```python
from build123d import *

# Parameters (mm, degrees)
F0_W      = 198
F0_H      = 198
F1_DEPTH  = 30
F2_W      = 138
F2_H      = 138
F3_DEPTH  = 30
F4_W      = 94
F4_H      = 94
F5_DEPTH  = 30
F6_R      = 4
F7_DEPTH  = 215
F9_DEPTH  = 215
F11_DEPTH = 25
F13_DEPTH = 25
F15_DEPTH = 25
F17_DEPTH = 25
F18_R     = 33.2568147927
F19_DEPTH = 6
F20_R     = 105
F20_R_2   = 33.2568147927
F21_DEPTH = 170
F21_TAPER = 10


with BuildPart() as f1:
    # F0 (on Top) → F1 (new body)
    with BuildSketch(Plane.XY):
        with Locations((99, 99)):
            Rectangle(F0_W, F0_H)
    extrude(amount=F1_DEPTH)

    # F2 (on face) → F3 (join)
    with BuildSketch(Plane.XY.offset(30)):
        with Locations((99, 99)):
            Rectangle(F2_W, F2_H)
    extrude(amount=F3_DEPTH)

    # F4 (on face) → F5 (join)
    with BuildSketch(Plane.XY.offset(60)):
        with Locations((99, 99)):
            Rectangle(F4_W, F4_H)
    extrude(amount=F5_DEPTH)

    # F6 (on face) → F7 (join)
    with BuildSketch(Plane.XY.offset(90)):
        with Locations((99, 99)):
            Circle(F6_R)
    extrude(amount=F7_DEPTH)

    # F8 (on face) → F9 (join)
    with BuildSketch(Plane.XY.offset(90)):
        Polygon((86.6256313292, 111.3743686708), (65.4124278936, 132.5875721064), (60.1091270347, 127.2842712475), (81.3223304703, 106.0710678119), align=None)
        Polygon((70.7157287525, 137.8908729653), (65.4124278936, 132.5875721064), (86.6256313292, 111.3743686708), (91.9289321881, 116.6776695297), align=None)
        Polygon((127.2842712475, 137.8908729653), (106.0710678119, 116.6776695297), (111.3743686708, 111.3743686708), (132.5875721064, 132.5875721064), align=None)
        Polygon((132.5875721064, 132.5875721064), (111.3743686708, 111.3743686708), (116.6776695297, 106.0710678119), (137.8908729653, 127.2842712475), align=None)
        Polygon((137.8908729653, 70.7157287525), (116.6776695297, 91.9289321881), (111.3743686708, 86.6256313292), (132.5875721064, 65.4124278936), align=None)
        Polygon((111.3743686708, 86.6256313292), (106.0710678119, 81.3223304703), (127.2842712475, 60.1091270347), (132.5875721064, 65.4124278936), align=None)
        Polygon((91.9289321881, 81.3223304703), (86.6256313292, 86.6256313292), (65.4124278936, 65.4124278936), (70.7157287525, 60.1091270347), align=None)
        Polygon((86.6256313292, 86.6256313292), (81.3223304703, 91.9289321881), (60.1091270347, 70.7157287525), (65.4124278936, 65.4124278936), align=None)
    extrude(amount=F9_DEPTH)

    # F10 (on face) → F11 (cut)
    with BuildSketch(Plane(origin=(5.3033008589, -5.3033008589, 0), x_dir=(0.7071067812, 0.7071067812, 0), z_dir=(0.7071067812, -0.7071067812, 0))):
        with BuildLine():
            Line((122.5071426749, 90), (122.5071426749, 305))
            ThreePointArc((122.5071426749, 305), (108.1413524776, 197.5), (122.5071426749, 90))
        make_face()
        with BuildLine():
            ThreePointArc((100.5295589566, 90), (93.5255146575, 197.840533222), (107.5071426749, 305))
            Line((107.5071426749, 305), (92.5071426749, 305))
            Line((92.5071426749, 305), (92.5071426749, 90))
            Line((92.5071426749, 90), (100.5295589566, 90))
        make_face()
    extrude(amount=-F11_DEPTH, mode=Mode.SUBTRACT)

    # F12 (on face) → F13 (cut)
    with BuildSketch(Plane(origin=(104.3033008589, 104.3033008589, 0), x_dir=(-0.7071067812, 0.7071067812, 0), z_dir=(0.7071067812, 0.7071067812, 0))):
        with BuildLine():
            Line((17.5, 305), (17.5, 90))
            ThreePointArc((17.5, 90), (28.9852035419, 197.5), (17.5, 305))
        make_face()
        with BuildLine():
            ThreePointArc((32.5, 305), (46.5125090054, 197.8568495491), (39.962310344, 90))
            Line((39.962310344, 90), (47.5, 90))
            Line((47.5, 90), (47.5, 305))
            Line((47.5, 305), (32.5, 305))
        make_face()
    extrude(amount=-F13_DEPTH, mode=Mode.SUBTRACT)

    # F14 (on face) → F15 (cut)
    with BuildSketch(Plane(origin=(5.3033008589, -5.3033008589, 0), x_dir=(0.7071067812, 0.7071067812, 0), z_dir=(0.7071067812, -0.7071067812, 0))):
        with BuildLine():
            ThreePointArc((172.5071426749, 305), (186.2558070406, 197.8608173435), (180.4356426001, 90))
            Line((180.4356426001, 90), (187.5071426749, 90))
            Line((187.5071426749, 90), (187.5071426749, 305))
            Line((187.5071426749, 305), (172.5071426749, 305))
        make_face()
        with BuildLine():
            Line((157.5071426749, 305), (157.5071426749, 90))
            ThreePointArc((157.5071426749, 90), (167.3211795092, 197.5), (157.5071426749, 305))
        make_face()
    extrude(amount=-F15_DEPTH, mode=Mode.SUBTRACT)

    # F16 (on face) → F17 (cut)
    with BuildSketch(Plane(origin=(104.3033008589, 104.3033008589, 0), x_dir=(-0.7071067812, 0.7071067812, 0), z_dir=(0.7071067812, 0.7071067812, 0))):
        with BuildLine():
            ThreePointArc((-42.129099369, 90), (-46.2365441061, 197.8995849807), (-32.5, 305))
            Line((-32.5, 305), (-47.5, 305))
            Line((-47.5, 305), (-47.5, 90))
            Line((-47.5, 90), (-42.129099369, 90))
        make_face()
        with BuildLine():
            Line((-17.5, 90), (-17.5, 305))
            ThreePointArc((-17.5, 305), (-27.2443014962, 197.5), (-17.5, 90))
        make_face()
    extrude(amount=-F17_DEPTH, mode=Mode.SUBTRACT)

    # F18 (on face) → F19 (join)
    with BuildSketch(Plane.XY.offset(305)):
        with Locations((99, 99)):
            Circle(F18_R)
    extrude(amount=F19_DEPTH)

    # F20 (on face) → F21 (join)
    with BuildSketch(Plane.XY.offset(311)):
        with Locations((99, 99)):
            Circle(F20_R)
        with Locations((99, 99)):
            Circle(F20_R_2, mode=Mode.SUBTRACT)
        with Locations((99, 99)):
            Circle(F20_R_2)
    extrude(amount=F21_DEPTH, taper=F21_TAPER)


solid = f1.part
```
Check sheet for the modelled part. Datum: model origin and axes. Units: mm. A direction names the side the tool comes from. Give positions to 0.01 mm unless a question says otherwise; leave off trailing zeros. Write each loop counter-clockwise with the first axis right and the second up, starting at its lowest first coordinate (ties: lowest second). Pieces come first, ordered by that corner, then holes. Notation, with made-up numbers: (41.25, 78.25) - (83.25, 78.25) arc R28 cw to (83.25, 102.25) - close; hole circle Ø4 at (-26, 47). An arc over 180 degrees is marked (long way). Answer as a JSON object with one key per item and string values. Group by question number.
1) Sectioned sample at A-A (z = 200). Record the cut outline in (x, y).
2) Access from +Z, -Z, +X, -X, +Y, -Y to the whole of each face (thin tool, end or side, straight path). Record for faces 4 (the face through (98, 146, 75)), 5 (the face through (0, 98, 15)), 6 (the face through (98, 52, 75)), 7 (the face through (76.54, 76.4, 199.02)).
3) Sectioned sample at B-B (z = 414). Record the cut outline in (x, y), then the cut area to 3 significant figures.
4) Release check for a two-part mould opening along Z. For faces 1 (the face through (198, 98, 15)), 2 (the face through (98, 100, 0)), 3 (the face through (68.817, 79.424, 195.995)) record: pulls with the +Z half, pulls with the -Z half, needs draft (parallel to the pull), parting line crosses it, or undercut.
5) Depth check by flat-ended pin: P1, Ø9, axis at y = 91, z = 68.5, coming from the +X side; P2, Ø4, axis at y = 124.5, z = 341.5, coming from the +X side; P3, Ø9, axis at y = 109.5, z = 42.5, coming from the -X side. Enter the tip coordinate at first touch or a pass-through.
6) Thickness scan on probe 1 along Z at (x, y) = (51.5, 137.5); probe 2 along Z at (x, y) = (63, 60.5); probe 3 along X at (y, z) = (108, 63). Record the ranges inside material, lowest first. Write a range as from..to.
Geometry results:
{
 "1": {"outline": "(60.86, 126.53) - (73.21, 114.19) - (83.81, 124.79) - (71.47, 137.14) - close; (60.88, 71.49) - (71.49, 60.88) - (81.78, 71.17) - (71.17, 81.78) - close; circle Ø8 at (99, 99); (112.96, 74.44) - (126.32, 61.07) - (136.93, 71.68) - (123.56, 85.04) - close; (113.01, 123.61) - (123.61, 113.01) - (136.95, 126.34) - (126.34, 136.95) - close"},
 "2": {"face 4": "+X, -X, +Y", "face 5": "-Z, -X, +Y, -Y", "face 6": "+X, -X, -Y", "face 7": "none"},
 "3": {"outline": "circle Ø173.68 at (99, 99)", "area": "23,700 mm^2"},
 "4": {"face 1": "needs draft", "face 2": "pulls with the -Z half", "face 3": "undercut"},
 "5": {"P1": "stops at x = 146", "P2": "stops at x = 195.93", "P3": "stops at x = 30"},
 "6": {"probe 1": "z = 0..60, 311..481", "probe 2": "z = 0..90, 311..481", "probe 3": "x = 52..146"}
}
